Source: CAD feature listing. Evaluate the final solid. Frame: model axes, mm. A direction names the side the tool comes from. Give positions to 0.01 mm unless a question says otherwise; leave off trailing zeros. Loops run counter-clockwise (first coordinate to the right, second up) from the corner with the lowest first, then second, coordinate; pieces in that order, holes last.
```python
from build123d import *

# Parameters (mm, degrees)
F0_W           = 65
F0_H           = 65
F1_DEPTH       = 10
F2_T           = -1
F6_DEPTH       = 10.0380592229
F6_DEPTH_BACK  = 30
F8_DEPTH       = 64.9
F8_DEPTH_BACK  = 36.001
F9_R           = 5
F10_DEPTH      = 25
F10_DEPTH_BACK = 1
F11_R          = 4
F12_DEPTH      = 1
F12_DEPTH_BACK = 22.5


with BuildPart() as f1:
    # F0 (on Top) → F1 (new body)
    with BuildSketch(Plane.XY):
        Rectangle(F0_W, F0_H)
    extrude(amount=F1_DEPTH)

    # F2
    f2_openings = [f1.faces().sort_by_distance(p)[0] for p in [
        (0, 0, 10),
    ]]
    offset(amount=F2_T, openings=f2_openings)

    # F5 (on face) → F6 (join, two sides)
    with BuildSketch(Plane(origin=(35.3553390593, -35.3553390593, 0), x_dir=(0.7071067812, 0.7071067812, 0), z_dir=(0.7071067812, -0.7071067812, 0))) as f6_sk:
        Polygon((6, 10), (5, 10), (5, 1), (-5, 1), (-5, 10), (-6, 10), (-6, 0), (6, 0), align=None)
    extrude(amount=-F6_DEPTH)
    extrude(f6_sk.sketch, amount=F6_DEPTH_BACK)

    # F7 (on face) → F8 (cut, two sides)
    with BuildSketch(Plane(origin=(35.3553390593, -35.3553390593, 0), x_dir=(0.7071067812, 0.7071067812, 0), z_dir=(0.7071067812, -0.7071067812, 0))) as f8_sk:
        Polygon((0, 10), (-5, 10), (-5, 1), (5, 1), (5, 10), align=None)
    extrude(amount=-F8_DEPTH, mode=Mode.SUBTRACT)
    extrude(f8_sk.sketch, amount=F8_DEPTH_BACK, mode=Mode.SUBTRACT)

    # F9 (on Top) → F10 (join, two sides)
    with BuildSketch(Plane.XY) as f10_sk:
        with Locations((49.8375721066, -49.8375721066)):
            Circle(F9_R)
    extrude(amount=-F10_DEPTH)
    extrude(f10_sk.sketch, amount=F10_DEPTH_BACK)

    # F11 (on Top) → F12 (cut, two sides)
    with BuildSketch(Plane.XY) as f12_sk:
        with Locations((49.8375721066, -49.8375721066)):
            Circle(F11_R)
    extrude(amount=F12_DEPTH, mode=Mode.SUBTRACT)
    extrude(f12_sk.sketch, amount=-F12_DEPTH_BACK, mode=Mode.SUBTRACT)


solid = f1.part
```
(1) Reachability of faces 1 (the flat face through (-5, -32.5, 5)), 2 (the flat face through (2, 32, 10)), 3 (the flat face through (32.5, 4, 5)), 4 (the flat face through (31.5, 3, 5)) from +Z, -Z, +X, -X, +Y, -Y: full face, straight path, thin tool, end or side. Return the list, or none.
A:
face 1: +Z, -Z, -X, -Y
face 2: +Z, +X, -X, +Y, -Y
face 3: +Z, -Z, +X, +Y
face 4: +Z
(2) Ray query, line 1 along Y through (x, z) = (16.5, 3); line 2 along Z through (x, y) = (-21, 24.5). Return the intervals inside material, ascending.
A:
line 1: y = -32.5 to -31.5, 31.5 to 32.5
line 2: z = 0 to 1
(3) Section D-D, the plane z = -16.5. Return the cut outline in (x, y).
A:
outline: circle Ø10 at (49.84, -49.84); hole circle Ø8 at (49.84, -49.84)
(4) Section A-A, the plane z = 5.5. Return the cut outline in (x, y).
A:
outline: (-32.5, -32.5) - (24.01, -32.5) - (52.33, -60.81) - (53.03, -60.1) - (24.43, -31.5) - (-31.5, -31.5) - (-31.5, 31.5) - (31.5, 31.5) - (31.5, -24.43) - (60.1, -53.03) - (60.81, -52.33) - (32.5, -24.01) - (32.5, 32.5) - (-32.5, 32.5) - close
(5) First-contact query: pin 1 (8 mm diameter, centred on x = 25.5, z = 5.5, fed in from -Y); pin 2 (7 mm diameter, centred on x = -12, z = 6.5, fed in from -Y); pin 3 (8 mm diameter, centred on y = 18, z = 3, fed in from +X). Flat tips, straight axial feed; report the tip coordinate or a pass-through.
A:
pin 1: stops at y = -37.99
pin 2: stops at y = -32.5
pin 3: stops at x = 32.5
(6) Mould query, pull axis X, two halves, no side actions, for faces 5 (the flat face through (0, 31.5, 5)), 6 (the cylindrical face through (52.145, -54.273, -12.325)), 7 (the flat face through (1, -2, 0)). Classes: pulls with the +X half, pulls with the -X half, needs draft (parallel to the pull), parting line crosses it, or undercut.
A:
face 5: undercut
face 6: parting line crosses it
face 7: needs draft
(7) Section B-B, the plane y = -11.5. Return the cut outline in (x, z).
A:
outline: (-32.5, 0) - (32.5, 0) - (32.5, 10) - (31.5, 10) - (31.5, 1) - (-31.5, 1) - (-31.5, 10) - (-32.5, 10) - close
